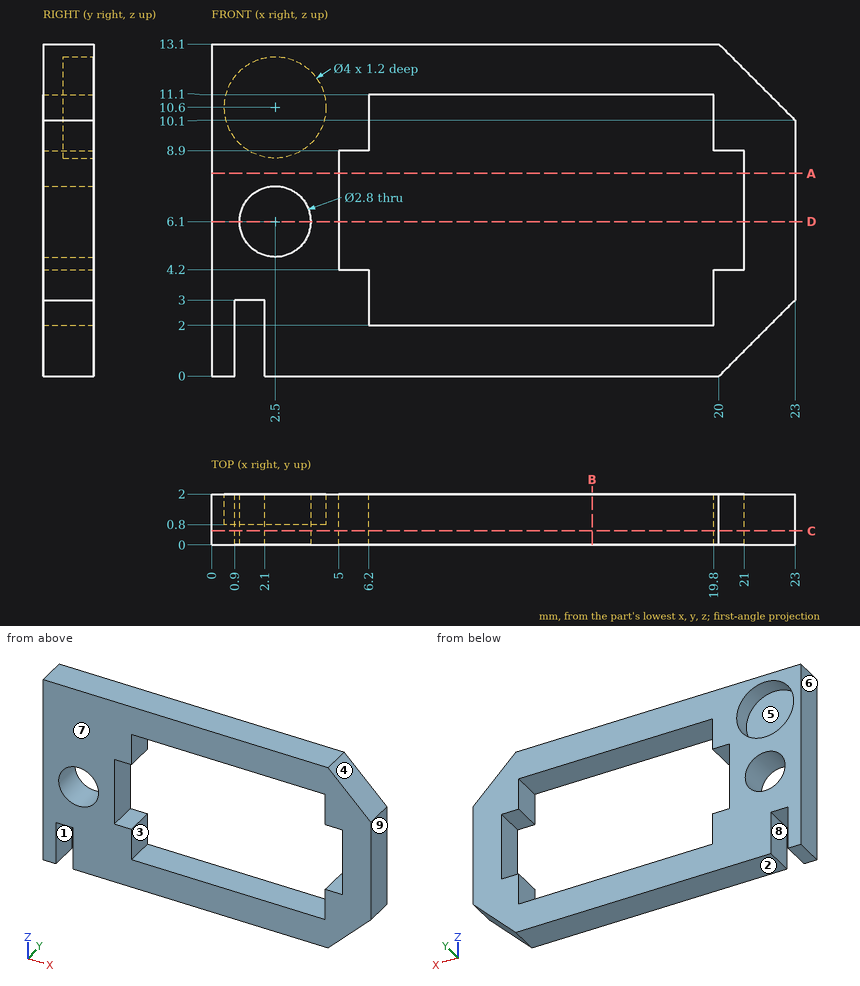
Geometry check sheet. Reference: drawing and pictorial views, mm from the part's lowest x, y, z. A direction names the side the tool comes from. Round coordinates to 2 decimals unless told otherwise and drop trailing zeros. Loops run counter-clockwise (first coordinate to the right, second up) from the corner with the lowest first, then second, coordinate; pieces in that order, holes last. Notation, with made-up numbers: (-22, -21.75) - (3, -21.75) arc R19 cw to (3, 6.25) - close; hole circle Ø3 at (-17, -17.75). An arc over 180 degrees is marked (long way). Write item = value, one per line. Start each with the question number.
Q1. Section check D-D (z = 6.1). Record the boundary of the cut face in (x, y).
Q2. Section check B-B (x = 15). Record the boundary of the cut face in (y, z), plus the area to 3 significant figures.
Q3. Access from +Z, -Z, +X, -X, +Y, -Y to the whole of each face (thin tool, end or side, straight path). Record for the marked faces 1, 2, 3, 4 and 5.
Q4. Release check for a two-part mould opening along X. For the marked faces 6, 7, 8 and 9 record: pulls with the +X half, pulls with the -X half, needs draft (parallel to the pull), parting line crosses it, or undercut.
Q5. Section check C-C (y = 0.55). Record the boundary of the cut face in (x, z), plus the area to 3 significant figures.
Q6. Section check A-A (z = 8). Record the boundary of the cut face in (x, y), plus the area to 3 significant figures.
Q7. Depth check by flat-ended pin: P1, Ø2.5, axis at x = 2.5, z = 6.1, coming from the +Y side. Enter the tip coordinate at first touch or a pass-through.
Q8. Thickness scan on L1, parallel to Z at x = 2.5, y = 1.45; L2, parallel to X at y = 1.1, z = 6.1; L3, parallel to X at y = 1.15, z = 7. Record the ranges inside material, lowest first.
Derived:
q1.outline = (0, 0) - (1.1, 0) - (1.1, 2) - (0, 2) - close; (3.9, 0) - (5, 0) - (5, 2) - (3.9, 2) - close; (21, 0) - (23, 0) - (23, 2) - (21, 2) - close
q2.outline = (0, 0) - (2, 0) - (2, 2) - (0, 2) - close; (0, 11.1) - (2, 11.1) - (2, 13.1) - (0, 13.1) - close
q2.area = 8.00 mm^2
q3.face_1 = -Z, +Y, -Y
q3.face_2 = -Z, +X, -X, +Y, -Y
q3.face_3 = +Y, -Y
q3.face_4 = +Z, +X, +Y, -Y
q3.face_5 = +Y
q4.face_6 = pulls with the -X half
q4.face_7 = needs draft
q4.face_8 = undercut
q4.face_9 = pulls with the +X half
q5.outline = (0, 0) - (0.9, 0) - (0.9, 3) - (2.1, 3) - (2.1, 0) - (20, 0) - (23, 3) - (23, 10.1) - (20, 13.1) - (0, 13.1) - close; hole circle Ø2.8 at (2.5, 6.1); hole (5, 4.2) - (6.2, 4.2) - (6.2, 2) - (19.8, 2) - (19.8, 4.2) - (21, 4.2) - (21, 8.9) - (19.8, 8.9) - (19.8, 11.1) - (6.2, 11.1) - (6.2, 8.9) - (5, 8.9) - close
q5.area = 148 mm^2
q6.outline = (0, 0) - (5, 0) - (5, 2) - (0, 2) - close; (21, 0) - (23, 0) - (23, 2) - (21, 2) - close
q6.area = 14.0 mm^2
q7.P1 = through
q8.L1 = 0 to 4.7, 7.5 to 8.6, 12.6 to 13.1
q8.L2 = 0 to 1.1, 3.9 to 5, 21 to 23
q8.L3 = 0 to 1.43, 3.57 to 5, 21 to 23
